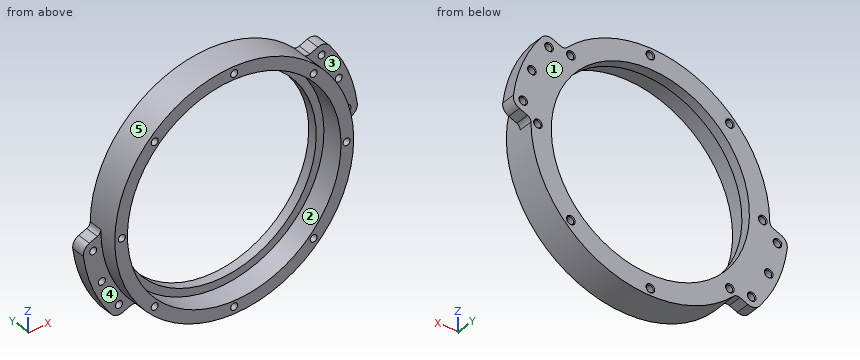
from build123d import *

# Parameters (mm, degrees)
SKETCH_1_R                   = 42.5
SKETCH_1_R_2                 = 38
EXTRUDE_1_DEPTH              = 11.5
EXTRUDE_START                = -3.5
SKETCH_2_R                   = 38
SKETCH_2_R_2                 = 35.25
EXTRUDE_2_DEPTH              = 3.5
SKETCH_3_R                   = 1
CUT_EXTRUDE_1_DEPTH          = 62.194362485
EXTRUDE_START_2              = -5
SKETCH_5_R                   = 1.15
EXTRUDE_3_DEPTH              = 5
FILLET_1_R                   = 2
HOLE_WIZARD_M3_1_D           = 2.5
HOLE_WIZARD_M3_1_CSINK_D     = 3.05
HOLE_WIZARD_M3_1_CSINK_ANGLE = 90
HOLE_WIZARD_M3_2_D           = 2.5
HOLE_WIZARD_M3_2_CSINK_D     = 3.05
HOLE_WIZARD_M3_2_CSINK_ANGLE = 90


with BuildPart() as part:
    # 草图1 → 凸台-拉伸1 (new body)
    with BuildSketch(Plane(origin=(0, 0, 0), x_dir=(1, 0, 0), z_dir=(0, 1, 0))):
        with Locations(Location((0, 0, 0), (0, 0, 270))):
            Circle(SKETCH_1_R)
        with Locations(Location((0, 0, 0), (0, 0, 270))):
            Circle(SKETCH_1_R_2, mode=Mode.SUBTRACT)
    extrude(amount=EXTRUDE_1_DEPTH)

    # 草图2 → 凸台-拉伸2 (add)
    with BuildSketch(Plane(origin=(0, 11.5, 0), x_dir=(1, 0, 0), z_dir=(0, 1, 0)).offset(EXTRUDE_START)):
        with Locations(Location((0, 0, 0), (0, 0, 270))):
            Circle(SKETCH_2_R)
        with Locations(Location((0, 0, 0), (0, 0, 270))):
            Circle(SKETCH_2_R_2, mode=Mode.SUBTRACT)
    extrude(amount=EXTRUDE_2_DEPTH)

    # 草图3 → 切除-拉伸1 (cut, through all)
    with BuildSketch(Plane.XZ):
        with Locations(Location((0, -40, 0), (0, 0, 270))):
            Circle(SKETCH_3_R)
        with Locations(Location((-28.284271247, -28.284271247, 0), (0, 0, 270))):
            Circle(SKETCH_3_R)
        with Locations(Location((-40, 0, 0), (0, 0, 270))):
            Circle(SKETCH_3_R)
        with Locations(Location((-28.284271247, 28.284271247, 0), (0, 0, 270))):
            Circle(SKETCH_3_R)
        with Locations(Location((0, 40, 0), (0, 0, 270))):
            Circle(SKETCH_3_R)
        with Locations(Location((28.284271247, 28.284271247, 0), (0, 0, 270))):
            Circle(SKETCH_3_R)
        with Locations(Location((40, 0, 0), (0, 0, 270))):
            Circle(SKETCH_3_R)
        with Locations(Location((28.284271247, -28.284271247, 0), (0, 0, 270))):
            Circle(SKETCH_3_R)
    extrude(amount=-CUT_EXTRUDE_1_DEPTH, mode=Mode.SUBTRACT)

    # 草图5 → 凸台-拉伸3 (add)
    # profile 1 of 2: a face of its own
    with BuildSketch(Plane(origin=(0, 11.5, 0), x_dir=(1, 0, 0), z_dir=(0, 1, 0)).offset(EXTRUDE_START_2)):
        with BuildLine():
            Line((34.719106229, -31.158203778), (30.628830889, -29.463956258))
            ThreePointArc((30.628830889, -29.463956258), (39.264880132, -16.264045876), (42.492017292, -0.82369075))
            Line((42.492017292, -0.82369075), (46.582292632, -2.51793827))
            ThreePointArc((46.582292632, -2.51793827), (48.270085945, -3.99477277), (48.714957389, -6.19290284))
            ThreePointArc((48.714957389, -6.19290284), (45.368967913, -18.79244182), (38.825720309, -30.067633122))
            ThreePointArc((38.825720309, -30.067633122), (36.956836015, -31.307374185), (34.719106229, -31.158203778))
        make_face()
        with Locations(Location((36.058498242, -27.924625414, 0), (0, 0, 270))):
            Circle(SKETCH_5_R, mode=Mode.SUBTRACT)
        with Locations(Location((45.242900619, -5.751516634, 0), (0, 0, 270))):
            Circle(SKETCH_5_R, mode=Mode.SUBTRACT)
        with Locations(Location((42.135389549, -17.453049807, 0), (0, 0, 270))):
            Circle(SKETCH_5_R, mode=Mode.SUBTRACT)
    # profile 2 of 2: a face of its own
    with BuildSketch(Plane(origin=(0, 11.5, 0), x_dir=(1, 0, 0), z_dir=(0, 1, 0)).offset(EXTRUDE_START_2)):
        with BuildLine():
            Line((-34.719106229, 31.158203778), (-30.628830889, 29.463956258))
            ThreePointArc((-30.628830889, 29.463956258), (-39.264880132, 16.264045876), (-42.492017292, 0.82369075))
            Line((-42.492017292, 0.82369075), (-46.582292632, 2.51793827))
            ThreePointArc((-46.582292632, 2.51793827), (-48.270085945, 3.99477277), (-48.714957389, 6.19290284))
            ThreePointArc((-48.714957389, 6.19290284), (-45.368967913, 18.79244182), (-38.825720309, 30.067633122))
            ThreePointArc((-38.825720309, 30.067633122), (-36.956836015, 31.307374185), (-34.719106229, 31.158203778))
        make_face()
        with Locations(Location((-36.058498242, 27.924625414, 0), (0, 0, 270))):
            Circle(SKETCH_5_R, mode=Mode.SUBTRACT)
        with Locations(Location((-45.242900619, 5.751516634, 0), (0, 0, 270))):
            Circle(SKETCH_5_R, mode=Mode.SUBTRACT)
        with Locations(Location((-42.135389549, 17.453049807, 0), (0, 0, 270))):
            Circle(SKETCH_5_R, mode=Mode.SUBTRACT)
    extrude(amount=EXTRUDE_3_DEPTH)

    # 圆角1
    fillet_1_edges = [part.edges().sort_by_distance(p)[0] for p in [
        (30.628830889, 9, 29.463956258),
        (42.492017292, 9, 0.82369075),
        (-30.628830889, 9, -29.463956258),
        (-42.492017292, 9, -0.82369075),
    ]]
    fillet(fillet_1_edges, radius=FILLET_1_R)

    # M3 螺纹孔1 (through all)
    with Locations(Plane(origin=(40, 11.5, 0), x_dir=(0, 0, 1), z_dir=(0, 1, 0))):
        with Locations((0, 0), (-28.284271247, -11.715728753), (-40, -40), (-28.284271247, -68.284271247), (0, -80), (28.284271247, -68.284271247), (17.453049807, 2.135389549), (5.751516634, 5.242900619), (-5.751516634, -85.242900619), (-17.453049807, -82.135389549), (-27.924625414, -76.058498242)):
            CounterSinkHole(HOLE_WIZARD_M3_1_D / 2, HOLE_WIZARD_M3_1_CSINK_D / 2, counter_sink_angle=HOLE_WIZARD_M3_1_CSINK_ANGLE)

    # M3 螺纹孔2 (through all)
    with Locations(Plane(origin=(36.058498242, 11.5, 27.924625414), x_dir=(0, 0, 1), z_dir=(0, 1, 0))):
        with Locations((0, 0), (0.359645833, -7.774226995), (12.075374586, -36.058498242)):
            CounterSinkHole(HOLE_WIZARD_M3_2_D / 2, HOLE_WIZARD_M3_2_CSINK_D / 2, counter_sink_angle=HOLE_WIZARD_M3_2_CSINK_ANGLE)


solid = part.part
Part model, mm, in its own coordinate system. Face numbers are marked on the shaded views. A direction names the side the tool comes from. Coordinates: 2 decimals unless noted, no trailing zeros. Order: outer loops, then holes, each group sorted by start corner. A loop starts at its lowest first (then second) coordinate and runs counter-clockwise, first axis right, second up.
(1) Slice it at B-B, the plane z = -13. Write the cut outline in (x, y), and give its area (3 significant figures).
Check sheet entries:
outline: (-47.36, 6.5) - (-40.46, 6.5) - (-40.46, 0) - (-35.71, 0) - (-35.71, 8) - (-32.77, 8) - (-32.77, 11.5) - (-47.36, 11.5) - close; (32.77, 8) - (35.71, 8) - (35.71, 0) - (40.46, 0) - (40.46, 11.5) - (32.77, 11.5) - close
area: 164 mm2
(2) Pin check, flat tips, straight feed: pin 1 Ø4 at (x, z) = (28.28, -28.28) entering from -Y; pin 2 Ø6 at (y, z) = (7.5, 23.5) entering from -X; pin 3 Ø6 at (x, y) = (13.5, 5) entering from +Z; pin 4 Ø1.5 at (y, z) = (9, 1) entering from +X. Stop position of each tip, or through.
Check sheet entries:
pin 1: stops at y = 0
pin 2: stops at x = -37.23
pin 3: stops at z = 41.18
pin 4: stops at x = 44.73
(3) Slice it at C-C, the plane y = 4. State how many separate pieces and enclosed holes the cut face has, and give its area (3 significant figures).
Check sheet entries:
separate pieces: 1
enclosed holes: 9
area: 1,100 mm2
(4) Pull direction X, two halves, no side cores. Call the marked faces 1 and 2: pulls with the +X half, pulls with the -X half, needs draft (parallel to the pull), parting line crosses it, or undercut.
Check sheet entries:
face 1: needs draft
face 2: undercut
(5) Probe L1, parallel to X at y = 5.75, z = 0; L2, parallel to X at y = 9, z = -17; L3, parallel to Z at x = 1, y = 3. List the from-to ranges inside material, lowest first.
Check sheet entries:
L1: x = -42.5 to -41.25, -38.75 to -38, 38 to 38.75, 41.25 to 42.5
L2: x = -46.07 to -43.3, -40.97 to -30.88, 30.88 to 38.95
L3: z = -42.49 to -40.75, -39.25 to -37.99, 37.99 to 39.25, 40.75 to 42.49
(6) Slice it at D-D, the plane x = 14.5. Write the cut outline in (y, z).
Check sheet entries:
outline: (0, -39.95) - (11.5, -39.95) - (11.5, -32.13) - (8, -32.13) - (8, -35.12) - (0, -35.12) - close; (0, 35.12) - (8, 35.12) - (8, 32.13) - (11.5, 32.13) - (11.5, 39.95) - (0, 39.95) - close
(7) Tool access for the marked faces 3, 4 and 5: list every direction of +Z, -Z, +X, -X, +Y, -Y with a clear straight run to the whole face (end or side of a thin tool).
Check sheet entries:
face 3: +Z, +X, -Y
face 4: -Z, -X, -Y
face 5: -Y
(8) Slice it at A-A, the plane x = 0. Write the cut outline in (y, z) (3 decimals), and give its area (3 significant figures).
Check sheet entries:
outline: (0, -42.5) - (11.5, -42.5) - (11.5, -41.525) - (11.225, -41.25) - (0, -41.25) - close; (0, -38.75) - (11.225, -38.75) - (11.5, -38.475) - (11.5, -35.25) - (8, -35.25) - (8, -38) - (0, -38) - close; (0, 38) - (8, 38) - (8, 35.25) - (11.5, 35.25) - (11.5, 38.475) - (11.225, 38.75) - (0, 38.75) - close; (0, 41.25) - (11.225, 41.25) - (11.5, 41.525) - (11.5, 42.5) - (0, 42.5) - close
area: 65.1 mm2
